from build123d import *

# Parameters (mm, degrees)
F0_W      = 17
F0_H      = 18
F1_DEPTH  = 10
F2_R      = 1.7
F3_DEPTH  = 25
F5_DEPTH  = 6.5
F7_DEPTH  = 6.5
F8_SIZE   = 5
F9_R      = 2
F11_DEPTH = 25
F12_R     = 5
F13_R     = 0.95
F14_DEPTH = 25
F15_R     = 0.875
F16_DEPTH = 25
F17_R     = 0.95
F18_DEPTH = 25


# Not quite as in the source:
# - a feature names something its author has since deleted; it is built from what else it names


with BuildPart() as f1:
    # F0 (on Front) → F1 (new body)
    with BuildSketch(Plane.XZ):
        Rectangle(F0_W, F0_H)
    extrude(amount=F1_DEPTH)

    # F2 (on face) → F3 (cut)
    with BuildSketch(Plane.XZ.offset(10)):
        Circle(F2_R)
    extrude(amount=-F3_DEPTH, mode=Mode.SUBTRACT)

    # F4 (on face) → F5 (cut)
    with BuildSketch(Plane(origin=(0, 0, -9), x_dir=(1, 0, 0), z_dir=(0, 0, -1))):
        Polygon((8.5, 10), (-8.5, 10), (-8.5, 7.002441328), align=None)
    extrude(amount=-F5_DEPTH, mode=Mode.SUBTRACT)

    # F6 (on face) → F7 (cut)
    with BuildSketch(Plane.XY.offset(9)):
        Polygon((8.5, -7.002441328), (-8.5, -10), (8.5, -10), align=None)
    extrude(amount=-F7_DEPTH, mode=Mode.SUBTRACT)

    # F8
    f8_edges = [f1.edges().sort_by_distance(p)[0] for p in [
        (0, 0, 9),
        (0, 0, -9),
    ]]
    chamfer(f8_edges, length=F8_SIZE)

    # F9
    f9_edges = [f1.edges().sort_by_distance(p)[0] for p in [
        (8.5, -8.501221, 2.5),
        (-8.5, -8.501221, -2.5),
        (8.5, -7.5, -9),
        (-8.5, -6.001221, -9),
        (8.5, -6.001221, 9),
        (-8.5, -7.5, 9),
    ]]
    fillet(f9_edges, radius=F9_R)

    # F10 (on face) → F11 (cut)
    with BuildSketch(Plane.XZ.offset(10)):
        Polygon((-8.5, -8), (-6, 0), (-8.5, 8), align=None)
        Polygon((8.5, -8), (8.5, 8), (6, 0), align=None)
    extrude(amount=-F11_DEPTH, mode=Mode.SUBTRACT)

    # F12
    f12_edges = [f1.edges().sort_by_distance(p)[0] for p in [
        (-6, -5, 0),
        (6, -5, 0),
    ]]
    fillet(f12_edges, radius=F12_R)

    # F13 (on face) → F14 (cut)
    with BuildSketch(Plane(origin=(1.453794355, -8.2448774948, 0), x_dir=(0.984807753, 0.1736481777, 0), z_dir=(0.1736481777, -0.984807753, 0))):
        with Locations((-1.3918819604, 5.9)):
            Circle(F13_R)
    extrude(amount=-F14_DEPTH, mode=Mode.SUBTRACT)

    # F15 (on face) → F16 (cut)
    with BuildSketch(Plane(origin=(-1.453794355, -8.2448774948, 0), x_dir=(0.984807753, -0.1736481777, 0), z_dir=(-0.1736481777, -0.984807753, 0))):
        with Locations((1.6190158435, -5.9)):
            Circle(F15_R)
    extrude(amount=-F16_DEPTH, mode=Mode.SUBTRACT)

    # F17 (on Right) → F18 (cut)
    with BuildSketch(Plane.YZ):
        with Locations((-5, 0)):
            Circle(F17_R)
    extrude(amount=-F18_DEPTH, mode=Mode.SUBTRACT)


solid = f1.part
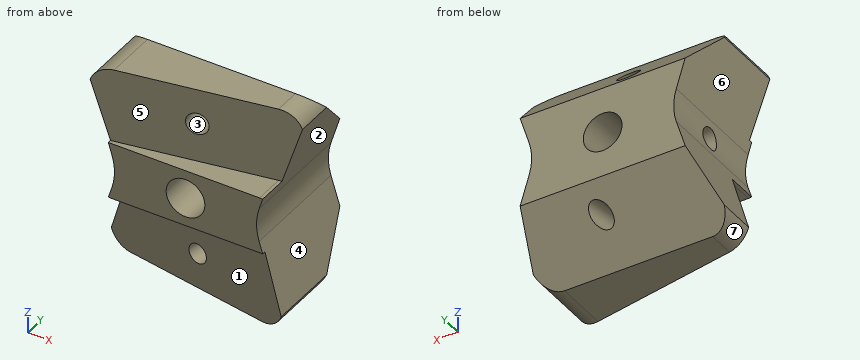
Build history of the part. All positions in model axes, mm. Face numbers are marked on the shaded views. A direction names the side the tool comes from. Round coordinates to 2 decimals unless told otherwise and drop trailing zeros. Write each loop counter-clockwise with the first axis right and the second up, starting at its lowest first coordinate (ties: lowest second). Pieces come first, ordered by that corner, then holes. Notation, with made-up numbers: M 70.25,-33.5 L 115.25,-33.5 A7 cw 115.25,-27.5 Z; hole C -23.5,48.25 d11. An arc over 180 degrees is marked long. Answer in a Markdown table with one row per item.
1. Saw through at D-D (x = 4). List the corners of the cut face in (y, z), and give its area (3 significant figures).
Geometry check:
| item | result |
|---|---|
| outline | M -10,-2.5 L -9.21,-2.5 L -9.21,-9 L -5,-9 L 0,-4 L 0,4 L -5,9 L -7.8,9 L -7.8,2.5 L -10,2.5 Z |
| area | 136 mm2 |
2. Probe L1, parallel to Y at x = -2.95, z = 0; L2, parallel to X at y = -3.75, z = 0; L3, parallel to X at y = -5.25, z = 6.25. List the from-to ranges inside material, lowest first. Write a range as [from, to].
Geometry check:
| item | result |
|---|---|
| L1 | [-10, -5.95], [-4.05, 0] |
| L2 | [-6.24, -1.7], [1.7, 6.24] |
| L3 | [-7.95, -1.38], [0.41, 7.95] |
3. Flat gauge pins, fed straight in: P1, Ø1.7, axis at y = -5, z = 0, coming from the -X side; P2, Ø6, axis at y = -3, z = -3, coming from the +X side (3 decimals); P3, Ø3, axis at x = 2, y = -2.5, coming from the +Z side; P4, Ø1.3, axis at x = -3, y = -8.5, coming from the -Z side. Where does each tip first touch, or does it go through?
Geometry check:
| item | result |
|---|---|
| P1 | x = 1.47 |
| P2 | x = 7.875 |
| P3 | z = 8 |
| P4 | z = -9 |
4. Mould opens along X. For the marked faces 1, 2 and 3 say: +X half, -X half, draft (parallel to the pull), parting line (faces both ways), or undercut.
Geometry check:
| item | result |
|---|---|
| face 1 | -X half |
| face 2 | +X half |
| face 3 | undercut |
5. Saw through at C-C (z = 1.25). List the corners of the cut face in (x, y), and give its area (3 significant figures).
Geometry check:
| item | result |
|---|---|
| outline | M -6.4,-10 L -1.15,-10 L -1.15,0 L -6.4,0 Z; M 1.15,-10 L 6.4,-10 L 6.4,0 L 1.15,0 Z |
| area | 105 mm2 |
6. Saw through at B-B (y = -9). List the corners of the cut face in (x, z).
Geometry check:
| item | result |
|---|---|
| outline | M -8.39,7.65 L -6.47,1.49 A5 cw -6.47,-1.49 L -6.78,-2.48 A2 ccw -6.5,-2.5 L 2.83,-2.5 L 2.83,-9 L 6.5,-9 A2 ccw 8.39,-7.65 L 6.47,-1.49 A5 cw 6.47,1.49 L 6.78,2.48 A2 ccw 6.5,2.5 L -2.83,2.5 L -2.83,9 L -6.5,9 A2 ccw Z; hole C 0,0 d3.4 |
7. Saw through at A-A (x = -3.75). List the corners of the cut face in (y, z).
Geometry check:
| item | result |
|---|---|
| outline | M -10,-2.5 L -7.84,-2.5 L -7.84,-9 L -5,-9 L 0,-4 L 0,4 L -5,9 L -9.16,9 L -9.16,2.5 L -10,2.5 Z; hole C -5,0 d1.9 |
8. Which spindle directions (+Z, -Z, +X, -X, +Y, -Y) get a long thin tool onto all of the face, cutting with end or side? Do the marked faces 4, 5, 6 and 7. Say none if no direction does.
Geometry check:
| item | result |
|---|---|
| face 4 | +X, +Y, -Y |
| face 5 | +Z, +X, -Y |
| face 6 | -X, +Y, -Y |
| face 7 | -Z, -X, +Y, -Y |
